from build123d import *

# Parameters (mm, degrees)
CROQUIS2_R                   = 2
SALIENTE_EXTRUIR1_DEPTH      = 20
CORTAR_EXTRUIR_L_MINA2_START = -0.6
CORTAR_EXTRUIR_L_MINA2_DEPTH = 0.6


# Read off the part's stored shape, not the designer's step: Cortar-Extruir-Lámina2
with BuildPart() as part:
    # Croquis2 → Saliente-Extruir1 (new body)
    with BuildSketch(Plane.XY):
        Circle(CROQUIS2_R)
    extrude(amount=-SALIENTE_EXTRUIR1_DEPTH)

    # Croquis4 → Revolución1 (revolve)
    with BuildSketch(Plane(origin=(0, 0, 0), x_dir=(1, 0, 0), z_dir=(0, 1, 0))):
        with BuildLine():
            Line((3.5, 20), (0, 20))
            Line((0, 20), (0, 22))
            ThreePointArc((0, 22), (2.015564437, 21.464737765), (3.5, 20))
        make_face()
    revolve(axis=Axis((0, 0, -20), (0, 0, -1)))

    # Cortar-Extruir-Lámina2 outline → Cortar-Extruir-Lámina2 (cut)
    with BuildSketch(Plane(origin=(0, 0, -22), x_dir=(-1, 0, 0), z_dir=(0, 0, -1)).offset(CORTAR_EXTRUIR_L_MINA2_START)):
        Polygon((0.1, -2), (0.1, -0.1), (2, -0.1), (2, 0.1), (0.1, 0.1), (0.1, 2), (-0.1, 2), (-0.1, 0.1), (-2, 0.1), (-2, -0.1), (-0.1, -0.1), (-0.1, -2), align=None)
    extrude(amount=CORTAR_EXTRUIR_L_MINA2_DEPTH, mode=Mode.SUBTRACT)


solid = part.part
For this review, take the finished solid that the model builds, in its own axes (mm). A direction names the side the tool comes from. Round coordinates to 2 decimals unless told otherwise and drop trailing zeros. Loops run counter-clockwise (first coordinate to the right, second up) from the corner with the lowest first, then second, coordinate; pieces in that order, holes last. Notation, with made-up numbers: (78.25, 74.5) - (123.25, 74.5) arc R9 cw to (123.25, 89.5) - close; hole circle Ø10 at (46, 45.5). An arc over 180 degrees is marked (long way). One line per item, written item: value. Start each with the question number.
Item 1: Take a section at C-C (z = -12.5). Give the boundary of the cut face in (x, y), plus the area to 3 significant figures.
Item 2: Clearance check with flat-ended pins moving along their axes: pin 1 Ø1 at (x, z) = (-2, -12.5) entering from +Y; pin 2 Ø1 at (x, z) = (0, -4) entering from -Y; pin 3 Ø0.5 at (x, z) = (0.5, -21.5) entering from +Y. State where each tip first meets the part, or that it passes through.
Item 3: Take a section at B-B (x = 1.75). Give the boundary of the cut face in (y, z).
Item 4: Take a section at D-D (y = 2.5). Give the boundary of the cut face in (x, z), plus the area to 3 significant figures.
Item 5: For faces 1 (the flat face through (2, 2, -20)), 2 (the flat face through (0, 0, 0)), list the 3-axis set-ups (+Z, -Z, +X, -X, +Y, -Y) from which the entire face can be reached by the end or side of a thin tool; tool diameter is ignored.
Item 6: For L1, parallel to Z at x = 1.5, y = 1.5; L2, parallel to Y at x = -1.5, z = -4.25; L3, parallel to X at y = 0.25, z = -8.25, list the stretches that pass through material, from the lowest coordinate up.
Answer below:
1. outline: circle Ø4 at (0, 0)
1. area: 12.6 mm2
2. pin 1: stops at y = 1.32
2. pin 2: stops at y = -2
2. pin 3: stops at y = 2.3
3. outline: (-3.03, -20) arc R3.67 ccw to (-0.1, -21.6) - (-0.1, -21.4) - (0.1, -21.4) - (0.1, -21.6) arc R3.67 ccw to (3.03, -20) - (0.97, -20) - (0.97, 0) - (-0.97, 0) - (-0.97, -20) - close
4. outline: (-2.45, -20) arc R3.2 ccw to (2.45, -20) - close
4. area: 3.88 mm2
5. face 1: +Z
5. face 2: +Z, +X, -X, +Y, -Y
6. L1: z = -21.4 to -20
6. L2: y = -1.32 to 1.32
6. L3: x = -1.98 to 1.98
